Could you check a few things on this model? Use its own coordinates, in mm. Give positions to 0.01 mm unless a question says otherwise; leave off trailing zeros. Loops run counter-clockwise (first coordinate to the right, second up) from the corner with the lowest first, then second, coordinate; pieces in that order, holes last. Notation, with made-up numbers: (12.25, 23.25) - (23.25, 23.25) arc R27 cw to (23.25, 51.25) - close; hole circle Ø10 at (24, -5). An arc over 180 degrees is marked (long way). Write each question's results on one line, items separated by ' | '. Start each with the question number.
1) If I drill on probe 1 along X at (y, z) = (5.5, 0); probe 2 along Z at (x, y) = (33.5, 1); probe 3 along X at (y, z) = (4, -32.5), over which ranges is the centre line in solid material (lowest first)? Write a range as [from, to].
2) I want a section at A-A, the plane x = -32.5. Write out the boundary of the cut face in (y, z), and give its area (3 significant figures).
3) I want a section at C-C, the plane y = 2. Count the separate pieces of the cut face and the enclosed holes in it, and give its area (3 significant figures).
4) I want a section at D-D, the plane x = -53. Write out the boundary of the cut face in (y, z), and give its area (3 significant figures).
5) I want a section at B-B, the plane z = 0. Write out the boundary of the cut face in (x, y), and give its area (3 significant figures).
from build123d import *

# Parameters (mm, degrees)
SKETCH1_W           = 130
SKETCH1_H           = 130
SKETCH1_R           = 25.5
SKETCH1_R_2         = 1.8
BOSS_EXTRUDE1_DEPTH = 7
FILLET1_R           = 10


with BuildPart() as part:
    # Sketch1 → Boss-Extrude1 (new body)
    with BuildSketch(Plane(origin=(0, 0, 0), x_dir=(1, 0, 0), z_dir=(0, 1, 0))):
        Rectangle(SKETCH1_W, SKETCH1_H)
        with Locations(Location((-32.5, 32.5, 0), (0, 0, 270))):
            Circle(SKETCH1_R, mode=Mode.SUBTRACT)
        with Locations(Location((32.5, 32.5, 0), (0, 0, 270))):
            Circle(SKETCH1_R, mode=Mode.SUBTRACT)
        with Locations(Location((-32.5, -32.5, 0), (0, 0, 270))):
            Circle(SKETCH1_R, mode=Mode.SUBTRACT)
        with Locations(Location((32.5, -32.5, 0), (0, 0, 270))):
            Circle(SKETCH1_R, mode=Mode.SUBTRACT)
        with Locations(Location((0, -53, 0), (0, 0, 270))):
            Circle(SKETCH1_R_2, mode=Mode.SUBTRACT)
        with Locations(Location((-53, 0, 0), (0, 0, 270))):
            Circle(SKETCH1_R_2, mode=Mode.SUBTRACT)
        with Locations(Location((0, 53, 0), (0, 0, 90))):
            Circle(SKETCH1_R_2, mode=Mode.SUBTRACT)
        with Locations(Location((53, 0, 0), (0, 0, 90))):
            Circle(SKETCH1_R_2, mode=Mode.SUBTRACT)
    extrude(amount=BOSS_EXTRUDE1_DEPTH)

    # Fillet1
    fillet1_edges = [part.edges().sort_by_distance(p)[0] for p in [
        (-65, 3.5, -65),
        (65, 3.5, -65),
        (65, 3.5, 65),
        (-65, 3.5, 65),
    ]]
    fillet(fillet1_edges, radius=FILLET1_R)


solid = part.part
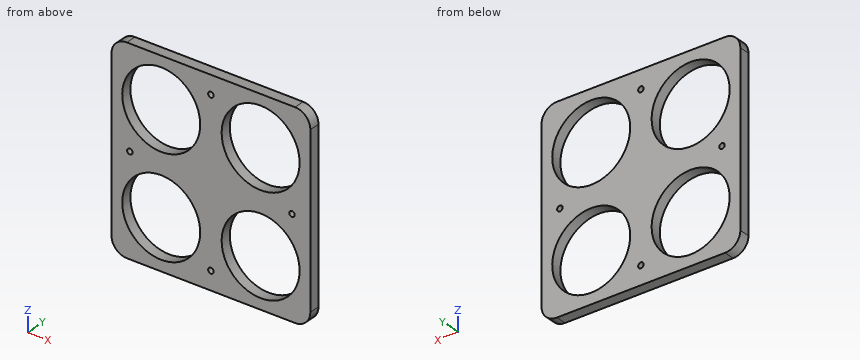
Answers:
1) probe 1: x = [-65, -54.8], [-51.2, 51.2], [54.8, 65] | probe 2: z = [-65, -57.98], [-7.02, 7.02], [57.98, 65] | probe 3: x = [-65, -58], [-7, 7], [58, 65]
2) outline: (0, -65) - (7, -65) - (7, -58) - (0, -58) - close; (0, -7) - (7, -7) - (7, 7) - (0, 7) - close; (0, 58) - (7, 58) - (7, 65) - (0, 65) - close | area: 196 mm2
3) separate pieces: 1 | enclosed holes: 8 | area: 8,600 mm2
4) outline: (0, -65) - (7, -65) - (7, -47.67) - (0, -47.67) - close; (0, -17.33) - (7, -17.33) - (7, -1.8) - (0, -1.8) - close; (0, 1.8) - (7, 1.8) - (7, 17.33) - (0, 17.33) - close; (0, 47.67) - (7, 47.67) - (7, 65) - (0, 65) - close | area: 460 mm2
5) outline: (-65, 0) - (-54.8, 0) - (-54.8, 7) - (-65, 7) - close; (-51.2, 0) - (51.2, 0) - (51.2, 7) - (-51.2, 7) - close; (54.8, 0) - (65, 0) - (65, 7) - (54.8, 7) - close | area: 860 mm2
